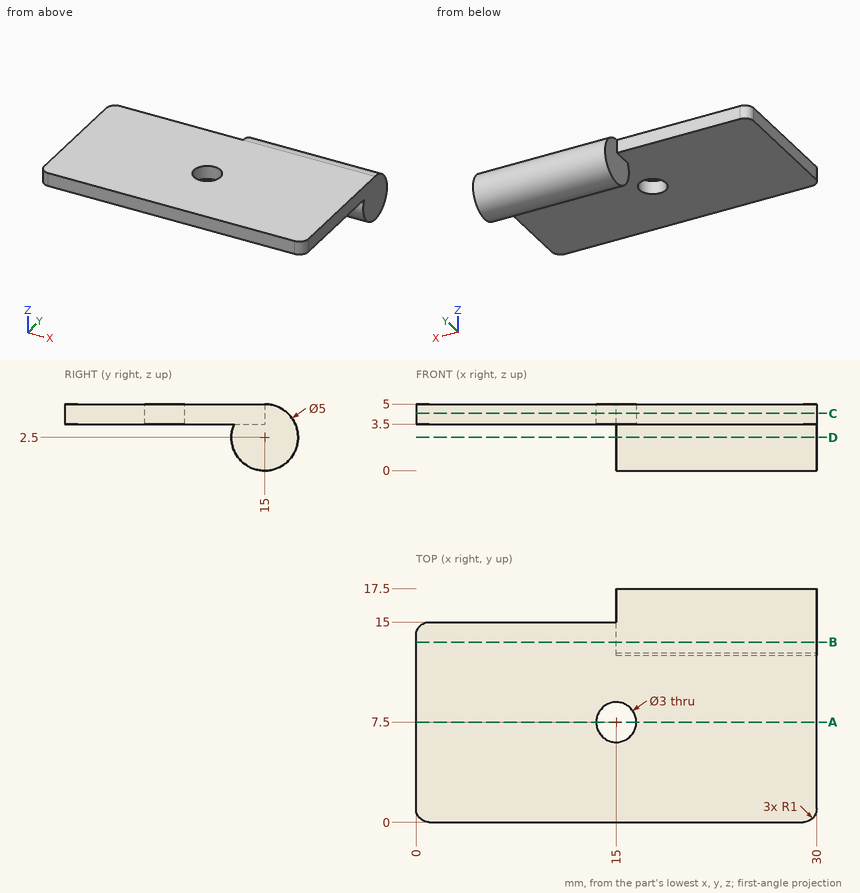
The drawing under review shows one solid part. Ordinate dimensions are in mm from its lowest x, y, z. Coordinates: 2 decimals unless noted, no trailing zeros. Order: outer loops, then holes, each group sorted by start corner. A loop starts at its lowest first (then second) coordinate and runs counter-clockwise, first axis right, second up. Notation, with made-up numbers: M -34.5,70.25 L -12.5,70.25 A16 ccw -12.5,79.25 Z; hole C -29,14.25 d6. An arc over 180 degrees is marked long. One line per question, with ' | ' between items.
(1) Add section A-A, the plane y = 7.5. Write out the cut boundary in (x, z), then the cut area to 3 significant figures.
Geometry results:
outline: M 0,3.5 L 13.5,3.5 L 13.5,5 L 0,5 Z; M 16.5,3.5 L 30,3.5 L 30,5 L 16.5,5 Z | area: 40.5 mm²
(2) Add section C-C, the plane z = 4.3. Write out the cut boundary in (x, y).
Geometry results:
outline: M 0,1 A1 ccw 1,0 L 29,0 A1 ccw 30,1 L 30,16.73 L 15,16.73 L 15,15 L 1,15 A1 ccw 0,14 Z; hole C 15,7.5 d3
(3) Insertion check: pin 1 (1.5 mm diameter, centred on y = 14, z = 1.5, fed in from -X); pin 2 (1.6 mm diameter, centred on x = 8, z = 4.5, fed in from +Y); pin 3 (2 mm diameter, centred on x = 16.5, z = 1, fed in from +Y). Each pin has a flat end and moves straight along its axis. Give the tip position at first contact, or say it passes through.
Geometry results:
pin 1: stops at x = 15 | pin 2: stops at y = 15 | pin 3: stops at y = 17.45
(4) Add section D-D, the plane z = 2.5. Write out the cut boundary in (x, y).
Geometry results:
outline: M 15,12.5 L 30,12.5 L 30,17.5 L 15,17.5 Z
(5) For probe 1 along Z at (x, y) = (19.5, 11.5); probe 2 along Y at (x, z) = (9.25, 4.5); probe 3 along X at (y, z) = (13.5, 1), list the stretches that pass through material, from the lowest coordinate up. Write a range as from..to.
Geometry results:
probe 1: z = 3.5..5 | probe 2: y = 0..15 | probe 3: x = 15..30
(6) Add section B-B, the plane y = 13.5. Write out the cut boundary in (x, z), then the cut area to 3 significant figures.
Geometry results:
outline: M 0,3.5 L 15,3.5 L 15,0.5 L 30,0.5 L 30,5 L 0,5 Z | area: 90.0 mm²
